Drawing for the job (mm, zero at the part's lowest x, y, z). A direction names the side the tool comes from. Coordinates: 2 decimals unless noted, no trailing zeros. Write each loop counter-clockwise with the first axis right and the second up, starting at its lowest first coordinate (ties: lowest second). Pieces come first, ordered by that corner, then holes. Notation, with made-up numbers: M 6.25,83 L 35.25,83 A18 ccw 35.25,112 Z; hole C 5,-32.5 d2. An arc over 180 degrees is marked long. Use a Markdown table: item, result. Add a question column.
Q1. Tool access for the marked faces 1, 2, 3 and 4: list every direction of +Z, -Z, +X, -X, +Y, -Y with a clear straight run to the whole face (end or side of a thin tool).
Q2. Pin check, flat tips, straight feed: pin 1 Ø1.5 at (x, y) = (6.5, 7) entering from -Z; pin 2 Ø4 at (x, z) = (6, 16) entering from +Y; pin 3 Ø1.7 at (x, z) = (4, 17.5) entering from -Y. Stop position of each tip, or through.
Q3. Wall check: L1, parallel to Z at x = 2, y = 2.25; L2, parallel to Z at x = 6.25, y = 1.25; L3, parallel to Y at x = 4, z = 9.75. Give the ranges that are in metal, low to high. Write a range as from..to.
Q4. Slice it at A-A on x = 4. Write the cut outline in (y, z).
Q5. Slice it at C-C on z = 5.5. Write the cut outline in (x, y), then the cut area to 3 significant figures.
Q6. Slice it at D-D on y = 7.75. Write the cut outline in (x, z).
Q7. Slice it at B-B on y = 6.75. Write the cut outline in (x, z).
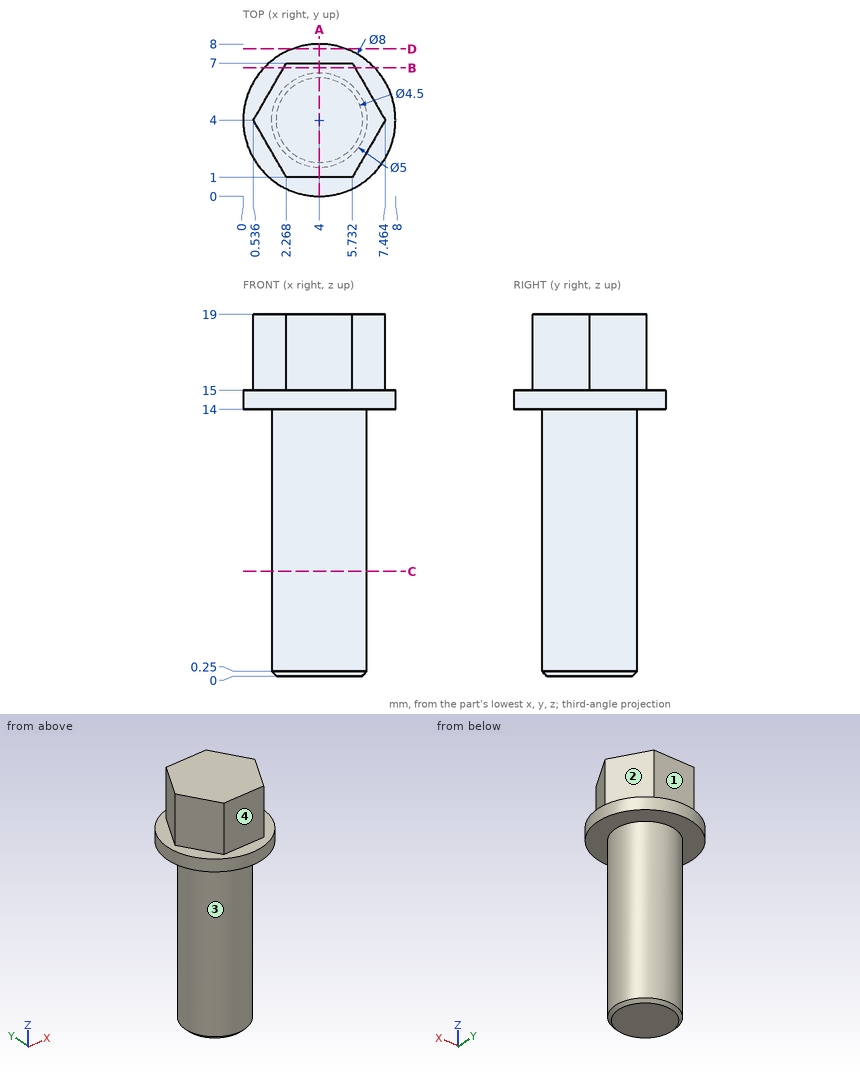
Recorded:
| question | item | result |
|---|---|---|
| 1 | face 1 | +Z, +X, -X, +Y |
| 1 | face 2 | +Z, +X, +Y |
| 1 | face 3 | -Z |
| 1 | face 4 | +Z, +X, -X, -Y |
| 2 | pin 1 | z = 14 |
| 2 | pin 2 | y = 7.99 |
| 2 | pin 3 | y = 1 |
| 3 | L1 | 14..19 |
| 3 | L2 | 14..15 |
| 3 | L3 | 1.5..6.5 |
| 4 | outline | M 0,14 L 1.5,14 L 1.5,0.25 L 1.75,0 L 6.25,0 L 6.5,0.25 L 6.5,14 L 8,14 L 8,15 L 7,15 L 7,19 L 1,19 L 1,15 L 0,15 Z |
| 5 | outline | C 4,4 d5 |
| 5 | area | 19.6 mm² |
| 6 | outline | M 2.61,14 L 5.39,14 L 5.39,15 L 2.61,15 Z |
| 7 | outline | M 1.1,14 L 6.9,14 L 6.9,15 L 5.88,15 L 5.88,19 L 2.12,19 L 2.12,15 L 1.1,15 Z |
